Autodesk Inventor part; units mm, degrees
ref_plane "YZ Plane" through (0, 0, 0) normal (1, 0, 0) x (0, 1, 0)
sketch "Sketch1" plane through (0, 0, 0) normal (0, 0, 1) x (1, 0, 0)
  arc A0 (6.35, 20.6311) -> (19.05, 20.6311) centre (12.7, 12.7) ccw
  circle A1 centre (12.7, 12.7) radius 8.255
  point P0 (0, 0)
  dimension "d0" = 16.51
extrude "Extrusion1" add sketch "Sketch1" against normal blind 50.8
ref_plane "Work Plane1" through (12.7, 20.955, 0) normal (0, 1, 0) x (-1, 0, 0)
sketch "Sketch2" plane through (12.7, 20.955, 0) normal (0, 1, 0) x (-1, 0, 0)
  line L0 (6.35, -15.875) -> (12.7, -15.875)
  line L1 (-12.7, -15.875) -> (-6.35, -15.875)
  line L2 (-6.35, -34.925) -> (-12.7, -34.925)
  line L3 (12.7, -34.925) -> (6.35, -34.925)
  line L4 (-8.255, -50.8) -> (8.255, -50.8)
  line L5 (-8.255, 0) -> (8.255, 0)
  line L6 (-6.4396, -15.875) -> (-6.4396, -34.925)
  line L7 (-6.4396, -34.925) -> (-6.4396, -25.4)
  line L8 (-6.4396, -34.925) -> (-6.4396, -30.1625)
  line L9 (6.4396, -15.875) -> (6.4396, -34.925)
  line L10 (6.4396, -25.4) -> (6.4396, -15.875)
  line L11 (6.4396, -20.6375) -> (6.4396, -15.875)
  line L12 (-6.4396, -32.5438) -> (6.4396, -32.5438)
  line L13 (6.4396, -32.5438) -> (6.4396, -18.2563)
  line L14 (6.4396, -18.2563) -> (-6.4396, -18.2563)
  line L15 (-6.4396, -18.2563) -> (-6.4396, -32.5438)
  point P0 (12.7, 0)
extrude "Extrusion2" add sketch "Sketch2" along normal blind 25.4 and the other way blind 8.255
chamfer "Chamfer1" distance 1.27 angle 45 2 edges at (12.7, 20.955, -18.2563) (12.7, 20.955, -32.5438)
sketch "Sketch3" plane through (12.7, 46.355, 0) normal (0, 1, 0) x (1, 0, 0)
  line L0 (6.4396, 32.5438) -> (-6.4396, 32.5438)
  line L1 (-6.4396, 32.5438) -> (-6.4396, 18.2563)
  line L2 (-6.4396, 18.2563) -> (6.4396, 18.2563)
  line L3 (6.4396, 18.2563) -> (6.4396, 32.5438)
  line L4 (-6.4396, 18.2563) -> (6.4396, 32.5438)
  line L5 (6.4396, 18.2563) -> (-6.4396, 32.5438)
  circle A0 centre (0, 25.4) radius 19.05
  circle A1 centre (0, 25.4) radius 13.97
  point P0 (-12.7, 0)
  dimension "d11" = 38.1
  dimension "d12" = 27.94
extrude "Extrusion3" add sketch "Sketch3" along normal blind 12.7 contours L4 L5 L0 | L3 L5 L4 | L5 L4 L1 | L2 L4 L5 | A1
extrude "Extrusion4" add sketch "Sketch3" along normal blind 31.75 contours A0
chamfer "Chamfer2" distance 10.16 angle 45 4 edges at (6.2604, 46.355, -25.4) (12.7, 46.355, -18.2563) (19.1396, 46.355, -25.4) (12.7, 46.355, -32.5438)
chamfer "Chamfer3" distance 2.54 angle 45 1 edges at (-6.35, 78.105, -25.4)
ref_plane "Work Plane2" through (4.445, 12.7, 0) normal (1, 0, 0) x (0, 1, 0)
sketch "Sketch4" plane through (19.1396, 17.8649, -16.9863) normal (1, 0, 0) x (0, 0, -1)
  line L0 (1.27, 18.3301) -> (15.5575, 18.3301)
  line L1 (1.27, 1.8534) -> (1.27, 18.3301)
  line L2 (16.8275, 0) -> (0, 0)
  line L3 (15.5575, 18.3301) -> (15.5575, 1.8534)
  line L4 (1.27, 1.8534) -> (15.5575, 1.8534)
  line L5 (8.4138, 1.8534) -> (8.4138, 4.3934)
  circle A0 centre (8.4138, 4.3934) radius 1.5875
  point P0 (-16.9863, -17.8649)
  dimension "d23" = 2.54
  dimension "d24" = 3.175
ref_plane "Work Plane3" through (19.1396, 17.8649, 0) normal (0.8660254, 0.5, 0) x (0, 0, 1)
sketch "Sketch5" plane through (19.1396, 17.8649, 0) normal (0.8660254, 0.5, 0) x (0, 0, 1)
  circle A0 centre (-25.4, -4.7625) radius 1.5875
  point P0 (0, 5.9017)
  dimension "d26" = 3.175
extrude "Extrusion5" cut sketch "Sketch5" along normal blind 12.7 and the other way blind 2.54
ref_plane "Work Plane4" through (12.7, 46.355, -6.35) normal (0, 0, 1) x (1, 0, 0)
sketch "Sketch6" plane through (12.7, 46.355, -6.35) normal (0, 0, 1) x (1, 0, 0)
  line L0 (16.5996, 0) -> (16.5996, 0)
  line L1 (16.5996, 0) -> (13.1137, -3.4859)
  arc A0 (13.1137, -3.4859) -> (7.9676, 0) centre (0, -17.3038) ccw
  line L2 (-7.9676, 0) -> (7.9676, 0)
  arc A1 (-7.9676, 0) -> (-13.1137, -3.4859) centre (0, -17.3038) ccw
  line L3 (-13.1137, -3.4859) -> (-16.5996, 0)
  line L4 (-16.5996, 0) -> (-16.5996, 0)
  line L5 (-16.5996, 0) -> (-13.1137, -3.4859)
  arc A2 (-7.9676, 0) -> (-13.1137, -3.4859) centre (0, -17.3038) ccw
  line L6 (7.9676, 0) -> (-7.9676, 0)
  arc A3 (13.1137, -3.4859) -> (7.9676, 0) centre (0, -17.3038) ccw
  line L7 (13.1137, -3.4859) -> (16.5996, 0)
  line L8 (19.05, 29.21) -> (-19.05, 29.21)
  line L9 (-19.05, 0) -> (-19.05, 29.21)
  line L10 (19.05, 0) -> (19.05, 29.21)
  line L11 (-19.05, 17.4625) -> (19.05, 17.4625)
  circle A4 centre (0, 17.4625) radius 1.5875
  point P0 (-12.7, -46.355)
  dimension "d31" = 3.175
hole "Hole1" at (12.7, 63.8175, -6.35) direction (0, 0, -1) diameter 3.175 end through all
ref_plane "Work Plane5" through (-240.4986, 445.264, 133.3441) normal (-0.8660254, -0.5, 0) x (-0.0199098, 0.0344847, -0.9992069)
sketch "Sketch7" plane through (-240.4986, 445.264, 133.3441) normal (-0.8660254, -0.5, 0) x (-0.0199098, 0.0344847, -0.9992069)
  circle A0 centre (25.4, -6.35) radius 1.5875
  point P0 (113.0953, 510.7677)
  dimension "d39" = 3.175
extrude "Extrusion6" cut sketch "Sketch7" against normal blind 12.7
properties part number "wrist-forearm"
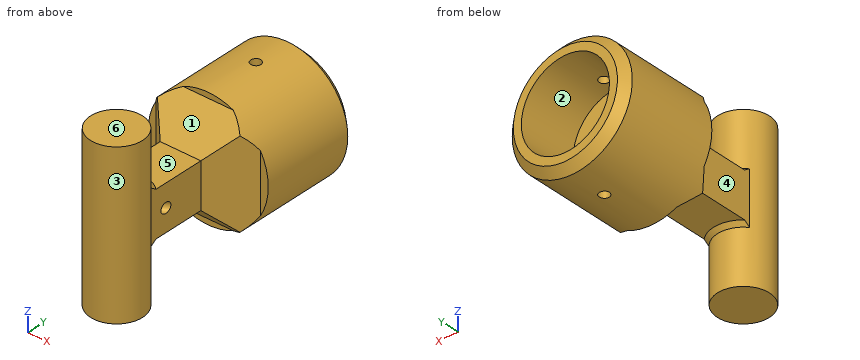
CAD build for the part. Positions are in the model's coordinates, mm. Face numbers are marked on the shaded views. A direction names the side the tool comes from. Coordinates: 2 decimals unless noted, no trailing zeros. Write each loop counter-clockwise with the first axis right and the second up, starting at its lowest first coordinate (ties: lowest second). Pieces come first, ordered by that corner, then holes. Notation, with made-up numbers: (48, 42) - (78, 42) arc R14 cw to (78, 48) - close; hole circle Ø9 at (-25, -35). An arc over 180 degrees is marked (long way). Use a Markdown table: item, result. Add a question column.
Item 1: Mould opens along Y. For the marked faces 4, 5 and 6 say: pulls with the +Y half, pulls with the -Y half, needs draft (parallel to the pull), parting line crosses it, or undercut.
Item 2: Band-saw the part on D-D, the plane y = 45. Give the cut face in (x, z).
Item 3: Band-saw the part on C-C, the plane z = -25.4. Give the cut face in (x, y) (3 decimals), and give its area (3 significant figures).
Item 4: Band-saw the part on B-B, the plane y = 67. Give the cut face in (x, z), and give its area (3 significant figures).
Item 5: Drill centre lines: L1, parallel to X at y = 65, z = -25; L2, parallel to X at y = 30.5, z = -27.5; L3, parallel to Z at x = 11, y = 25.5. Where is each one in solid material? Low to high. Write a range as from..to.
Item 6: 3-axis set-ups, long thin cutter, end or side, ignore diameter. For the marked faces 1, 2 and 3: which of +Z, -Z, +X, -X, +Y, -Y reach the whole face in a straight line?
Item 7: Band-saw the part on A-A, the plane x = 12.7. Give the number of separate pieces and of enclosed holes in the cut face, and give its area (3 significant figures).
Item 8: Flat gauge pins, fed straight in: pin 1 (1 mm diameter, centred on x = 8, y = 56.5, fed in from -Z); pin 2 (0.9 mm diameter, centred on x = 14, z = -7, fed in from -Y); pin 3 (4 mm diameter, centred on y = 59.5, z = -6.5, fed in from +X). Where does each tip first touch, or does it go through?
Numbers:
| question | item | result |
|---|---|---|
| 1 | face 4 | undercut |
| 1 | face 5 | undercut |
| 1 | face 6 | needs draft |
| 2 | outline | (-2.54, -36.82) arc R19.05 ccw to (2.28, -41.35) - (23.12, -41.35) arc R19.05 ccw to (27.94, -36.82) - (27.94, -13.98) arc R19.05 ccw to (23.12, -9.45) - (2.28, -9.45) arc R19.05 ccw to (-2.54, -13.98) - close |
| 3 | outline | (-6.35, 46.355) - (-3.9, 46.355) - (6.26, 36.195) - (6.26, 17.865) arc R8.255 ccw (long way) to (19.14, 17.865) - (19.14, 21.531) - (15.351, 19.344) - (13.763, 22.093) - (19.14, 25.197) - (19.14, 36.195) - (29.3, 46.355) - (31.75, 46.355) - (31.75, 75.565) - (29.21, 78.105) - (26.67, 78.105) - (26.67, 59.055) - (-1.27, 59.055) - (-1.27, 78.105) - (-3.81, 78.105) - (-6.35, 75.565) - close |
| 3 | area | 1,310 mm2 |
| 4 | outline | circle Ø38.1 at (12.7, -25.4); hole circle Ø27.94 at (12.7, -25.4) |
| 4 | area | 527 mm2 |
| 5 | L1 | -6.35..-1.26, 26.66..31.75 |
| 5 | L2 | 6.26..19.14 |
| 5 | L3 | -32.54..-18.26 |
| 6 | face 1 | +Z, +X, -X |
| 6 | face 2 | +Y |
| 6 | face 3 | none |
| 7 | separate pieces | 3 |
| 7 | enclosed holes | 0 |
| 7 | area | 1,950 mm2 |
| 8 | pin 1 | z = -43.98 |
| 8 | pin 2 | y = 4.49 |
| 8 | pin 3 | x = 21.49 |
